```python
from build123d import *

# Parameters (mm, degrees)
F0_W      = 342.9
F0_H      = 266.7
F1_DEPTH  = 25.4
F2_W      = 114.3
F2_H      = 215.9
F3_DEPTH  = 25.4
F4_W      = 12.7
F4_H      = 215.9
F5_DEPTH  = 19.05
F6_W      = 12.7
F6_H      = 215.9
F7_DEPTH  = 19.05
F9_W      = 330.2
F9_H      = 6.35
F10_DEPTH = 6.35
F11_W     = 6.35
F11_H     = 196.85
F12_DEPTH = 6.35


# Not quite as in the source:
# - a feature names something its author has since deleted; it is built from what else it names


with BuildPart() as f1:
    # F0 (on Front) → F1 (new body)
    with BuildSketch(Plane.XZ):
        with Locations((-171.45, 133.35)):
            Rectangle(F0_W, F0_H)
    extrude(amount=F1_DEPTH)

    # F2 (on face) → F3 (cut)
    with BuildSketch(Plane(origin=(0, 0, 0), x_dir=(-1, 0, 0), z_dir=(0, 1, 0))):
        with Locations((228.6, 107.95)):
            Rectangle(F2_W, F2_H)
        with Locations((114.3, 107.95)):
            Rectangle(F2_W, F2_H)
    extrude(amount=-F3_DEPTH, mode=Mode.SUBTRACT)

    # F4 (on face) → F5 (join)
    with BuildSketch(Plane.YZ.offset(-285.75)):
        with Locations((-19.05, 107.95)):
            Rectangle(F4_W, F4_H)
    extrude(amount=F5_DEPTH)

    # F6 (on face) → F7 (join)
    with BuildSketch(Plane(origin=(-57.15, 0, 0), x_dir=(0, -1, 0), z_dir=(-1, 0, 0))):
        with Locations((19.05, 107.95)):
            Rectangle(F6_W, F6_H)
    extrude(amount=F7_DEPTH)

    # F9 (on face) → F10 (cut)
    with BuildSketch(Plane.XZ.offset(25.4)):
        with Locations((-171.45, 260.35)):
            Rectangle(F9_W, F9_H)
    extrude(amount=-F10_DEPTH, mode=Mode.SUBTRACT)

    # F11 (on face) → F12 (cut)
    with BuildSketch(Plane.XZ.offset(25.4)):
        with Locations((-336.55, 123.825)):
            Rectangle(F11_W, F11_H)
        with Locations((-6.35, 123.825)):
            Rectangle(F11_W, F11_H)
    extrude(amount=-F12_DEPTH, mode=Mode.SUBTRACT)


solid = f1.part
```
Model file for the job. Use its own axes, mm. A direction names the side the tool comes from. Give positions to 0.01 mm unless a question says otherwise; leave off trailing zeros. Order: outer loops, then holes, each group sorted by start corner. A loop starts at its lowest first (then second) coordinate and runs counter-clockwise, first axis right, second up.
1) Pin check, flat tips, straight feed: pin 1 (3 mm diameter, centred on y = -21, z = 94.5, fed in from +X); pin 2 (3 mm diameter, centred on x = -221.5, y = -14, fed in from -Z). Stop position of each tip, or through.
2) Saw through at C-C, the plane y = -4.5. Write the cut outline in (x, z), then the cut area to 3 significant figures.
3) 3-axis set-ups, long thin cutter, end or side, ignore diameter. For faces 4 (the flat face through (-169, -25.4, 220)), 5 (the flat face through (-276, -12.7, 106)), 6 (the flat face through (-76.2, -19, 109)): which of +Z, -Z, +X, -X, +Y, -Y reach the whole face in a straight line?
4) Saw through at A-A, the plane z = 89. Write the cut outline in (x, y) (3 decimals), then the cut area to 3 significant figures.
5) Mould opens along X. For faces 1 (the flat face through (-342.9, -13, 131)), 2 (the flat face through (-173, -13, 215.9)), 3 (the flat face through (-305, -13, 0)) say: +X half, -X half, draft (parallel to the pull), parting line (faces both ways), or undercut.
6) Saw through at B-B, the plane x = -167. Write the cut outline in (y, z) (3 decimals), then the cut area to 3 significant figures.
7) Wall check: probe 1 along X at (y, z) = (-22.75, 205.5) (3 decimals); probe 2 along X at (y, z) = (-2, 209); probe 3 along Z at (x, y) = (-266, -22.5) (3 decimals). Give the ranges that are in metal, low to high.
Computed:
1. pin 1: stops at x = 0
1. pin 2: stops at z = 215.9
2. outline: (-342.9, 0) - (-285.75, 0) - (-285.75, 215.9) - (-57.15, 215.9) - (-57.15, 0) - (0, 0) - (0, 266.7) - (-342.9, 266.7) - close
2. area: 42,100 mm2
3. face 4: +Z, -Z, +X, -X, -Y
3. face 5: -Z, +Y
3. face 6: -Z, +Y, -Y
4. outline: (-342.9, -25.4) - (-339.725, -25.4) - (-339.725, -19.05) - (-333.375, -19.05) - (-333.375, -25.4) - (-266.7, -25.4) - (-266.7, -12.7) - (-285.75, -12.7) - (-285.75, 0) - (-342.9, 0) - close; (-76.2, -25.4) - (-9.525, -25.4) - (-9.525, -19.05) - (-3.175, -19.05) - (-3.175, -25.4) - (0, -25.4) - (0, 0) - (-57.15, 0) - (-57.15, -12.7) - (-76.2, -12.7) - close
4. area: 3,310 mm2
5. face 1: -X half
5. face 2: undercut
5. face 3: draft
6. outline: (-25.4, 215.9) - (0, 215.9) - (0, 266.7) - (-25.4, 266.7) - (-25.4, 263.525) - (-19.05, 263.525) - (-19.05, 257.175) - (-25.4, 257.175) - close
6. area: 1,250 mm2
7. probe 1: x = -342.9 to -339.725, -333.375 to -266.7, -76.2 to -9.525, -3.175 to 0
7. probe 2: x = -342.9 to -285.75, -57.15 to 0
7. probe 3: z = 215.9 to 257.175, 263.525 to 266.7
